Design review of the part built by this model. Coordinates are the model's own, in mm. Face numbers are marked on the shaded views. A direction names the side the tool comes from. Give positions to 0.01 mm unless a question says otherwise; leave off trailing zeros. Loops run counter-clockwise (first coordinate to the right, second up) from the corner with the lowest first, then second, coordinate; pieces in that order, holes last.
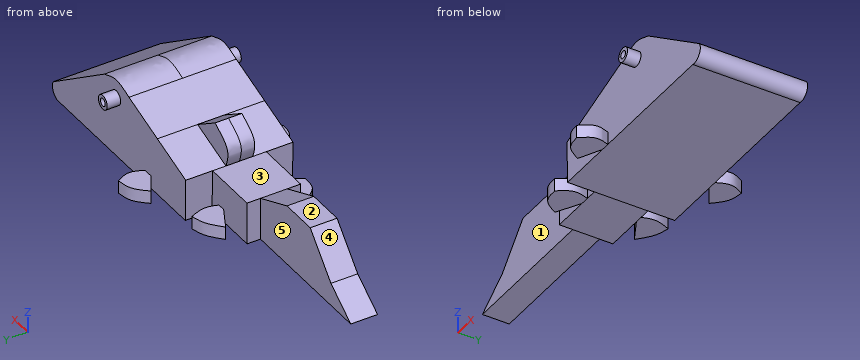
from build123d import *

# Parameters (mm, degrees)
F0_R     = 0.8499357061
F1_DEPTH = 6.35
F2_DEPTH = 3.175
F3_DEPTH = 1.5875
F4_DEPTH = 1.5875
F0_R_2   = 0.4591365961
F5_DEPTH = 7.9375
F6_DEPTH = 6.35
F9_DEPTH = 1.524


with BuildPart() as f1:
    # F0 (on Front) → F1 (new body, symmetric)
    with BuildSketch(Plane.XZ):
        with BuildLine():
            Line((3.7369009076, -7.1760629105), (27.8668981838, -7.1645976751))
            ThreePointArc((27.8668981838, -7.1645976751), (29.0924289966, -6.6745059956), (29.1452982829, -5.3556730016))
            Line((29.1452982829, -5.3556730016), (19.3140551537, 1.5164437805))
            add(Edge.make_bspline(
                [(19.3140551537, 1.5164437805), (18.5598178705, 1.842624393), (17.0255294285, 2.5061492361), (15.3991179845, 1.8500253214), (14.5722303488, 1.5164437805)],
                knots=[0, 0, 0, 0, 0.4915876753, 1, 1, 1, 1], degree=3))
            Line((14.5722303488, 1.5164437805), (9.1069049254, -0.31865054))
            Line((9.1069049254, -0.31865054), (3.641579502, -2.1537448606))
            Line((3.641579502, -2.1537448606), (3.7369009076, -7.1760629105))
        make_face()
        with Locations((17.0290809923, 0)):
            Circle(F0_R, mode=Mode.SUBTRACT)
    extrude(amount=F1_DEPTH, both=True)

    # F0 (on Front) → F2 (join, symmetric)
    with BuildSketch(Plane.XZ):
        Polygon((-3.0088014841, -7.1792680938), (3.7369009076, -7.1760629105), (3.641579502, -2.1537448606), (-2.9932308073, -2.1537448606), align=None)
    extrude(amount=F2_DEPTH, both=True)

    # F0 (on Front) → F3 (join, symmetric)
    with BuildSketch(Plane.XZ):
        Polygon((-20.3930963686, -7.1875281459), (-3.0088014841, -7.1792680938), (-2.9932308073, -2.1537448606), (-8.1067462721, 0), (-12.5872229892, 0), (-16.5754726262, -4.4647546742), align=None)
    extrude(amount=F3_DEPTH, both=True)

    # F0 (on Front) → F4 (join, symmetric)
    with BuildSketch(Plane.XZ):
        with BuildLine():
            add(Edge.make_bspline(
                [(5.739697431, 1.9025673836), (4.7061257381, 1.3267304785), (2.7990985393, 0.2642627845), (3.3769243884, -1.3941566443), (3.641579502, -2.1537448606)],
                knots=[0, 0, 0, 0, 0.5419806321, 1, 1, 1, 1], degree=3))
            Line((3.641579502, -2.1537448606), (9.1069049254, -0.31865054))
            Line((9.1069049254, -0.31865054), (5.739697431, 1.9025673836))
        make_face()
    extrude(amount=F4_DEPTH, both=True)

    # F0 (on Front) → F5 (join, symmetric)
    with BuildSketch(Plane.XZ):
        with Locations((17.0290809923, 0)):
            Circle(F0_R)
        with Locations((17.0290809923, 0)):
            Circle(F0_R_2, mode=Mode.SUBTRACT)
    extrude(amount=F5_DEPTH, both=True)

    # F0 (on Front) → F6 (join, symmetric)
    with BuildSketch(Plane.XZ):
        with Locations((17.0290809923, 0)):
            Circle(F0_R_2)
    extrude(amount=F6_DEPTH, both=True)

    # F8 (on offset) → F9 (join)
    with BuildSketch(Plane(origin=(0.0034105097, 0, -7.1778368579), x_dir=(0.9999998871, 0, 0.0004751444), z_dir=(0.0004751444, 0, -0.9999998871))):
        with BuildLine():
            Line((10.5719827116, 6.2902872451), (11.4731285721, 6.2886215746))
            add(Edge.make_bspline(
                [(11.4731285721, 6.2886215746), (11.6881530578, 6.8505612185), (12.1330545046, 8.0132553954), (11.2921062686, 9.0884414112), (10.8575951308, 9.6439812332)],
                knots=[0, 0, 0, 0, 0.483308128, 1, 1, 1, 1], degree=3))
            add(Edge.make_bspline(
                [(10.8575951308, 9.6439812332), (10.2459421425, 9.6264263255), (8.9601619026, 9.5895234992), (8.2060067921, 8.3258092197), (7.8106075525, 7.6632509008)],
                knots=[0, 0, 0, 0, 0.4757056489, 1, 1, 1, 1], degree=3))
            Line((7.8106075525, 7.6632509008), (10.5719827116, 6.2902872451))
        make_face()
        with BuildLine():
            add(Edge.make_bspline(
                [(11.445928365, -6.2551540323), (11.7208028901, -6.8377598255), (12.2652189582, -7.9916679237), (11.6289449799, -9.0578690758), (11.3139245659, -9.5857474953)],
                knots=[0, 0, 0, 0, 0.5048979368, 1, 1, 1, 1], degree=3))
            Line((11.445928365, -6.2551540323), (10.5652892962, -6.2281796709))
            Line((10.5652892962, -6.2281796709), (8.0862324685, -7.7491207048))
            add(Edge.make_bspline(
                [(11.3139245659, -9.5857474953), (10.7293926361, -9.5187590976), (9.5019236971, -9.3780889543), (8.572864944, -8.3090653448), (8.0862324685, -7.7491207048)],
                knots=[0, 0, 0, 0, 0.4762091973, 1, 1, 1, 1], degree=3))
        make_face()
        with BuildLine():
            add(Edge.make_bspline(
                [(2.4012238719, -3.135364037), (2.5766554897, -3.6317241258), (2.9495824062, -4.6868706955), (2.4212189682, -5.9031792319), (2.1414074581, -6.5473141149)],
                knots=[0, 0, 0, 0, 0.4704182467, 1, 1, 1, 1], degree=3))
            Line((2.4012238719, -3.135364037), (1.5678445343, -3.1441783067))
            Line((1.5678445343, -3.1441783067), (-1.2165163644, -4.6103880741))
            add(Edge.make_bspline(
                [(2.1414074581, -6.5473141149), (1.5835583581, -6.4193566225), (0.3958954029, -6.1469346133), (-0.6577640532, -5.1428505543), (-1.2165163644, -4.6103880741)],
                knots=[0, 0, 0, 0, 0.4697032587, 1, 1, 1, 1], degree=3))
        make_face()
        with BuildLine():
            Line((1.3515800238, 3.1687226146), (2.3737214506, 3.1360480934))
            add(Edge.make_bspline(
                [(2.3737214506, 3.1360480934), (2.5897819708, 3.7493472374), (3.0287531003, 4.9953902449), (2.2088825996, 6.1050612637), (1.792550087, 6.6685550846)],
                knots=[0, 0, 0, 0, 0.4921974706, 1, 1, 1, 1], degree=3))
            add(Edge.make_bspline(
                [(1.792550087, 6.6685550846), (1.1529153889, 6.6804914863), (-0.1895757498, 6.7055440354), (-0.9754613011, 5.3946395707), (-1.3869088143, 4.7083199024)],
                knots=[0, 0, 0, 0, 0.4764535334, 1, 1, 1, 1], degree=3))
            Line((-1.3869088143, 4.7083199024), (1.3515800238, 3.1687226146))
        make_face()
    extrude(amount=-F9_DEPTH)


solid = f1.part
Q1. Tool access review of the marked faces 1 and 2: name each direction out of +Z, -Z, +X, -X, +Y, -Y from which nothing blocks a thin tool from reaching the whole face with its end or side.
Results:
face 1: +Z, -Z, -X, -Y
face 2: +Z, -X, +Y, -Y
Q2. Take a section at B-B (x = 21.5). Give the boundary of the cut face in (y, z).
Results:
outline: (-6.35, -7.17) - (6.35, -7.17) - (6.35, -0.01) - (-6.35, -0.01) - close
Q3. Draft analysis for pull direction X (two halves, no side actions). For the marked faces 3, 4 and 5, state which applies: pulls with the +X half, pulls with the -X half, needs draft (parallel to the pull), parting line crosses it, or undercut.
Results:
face 3: undercut
face 4: pulls with the -X half
face 5: needs draft
Q4. Insertion check: pin 1 (4 mm diameter, centred on x = 2.5, z = -4, fed in from -Y); pin 2 (5 mm diameter, centred on x = 15.5, z = -2, fed in from +Y); pin 3 (3 mm diameter, centred on x = 7, z = 0.5, fed in from -Y). Each pin has a flat end and moves straight along its axis. Give the tip position at first contact, or say it passes through.
Results:
pin 1: stops at y = -6.67
pin 2: stops at y = 7.94
pin 3: stops at y = -6.35
Q5. Wall thickness on line 1 (Z direction, x = 11, y = 8.5); line 2 (Y direction, x = -17, z = -5.5); line 3 (Z direction, x = 1, y = 5.5): over which ranges is each line inside the solid? List them lowest first.
Results:
line 1: z = -7.17 to -5.65
line 2: y = -1.59 to 1.59
line 3: z = -7.18 to -5.65
Q6. Take a section at A-A (x = -5). Give the boundary of the cut face in (y, z), plus the area to 3 significant figures.
Results:
outline: (-1.59, -7.18) - (1.59, -7.18) - (1.59, -1.31) - (-1.59, -1.31) - close
area: 18.6 mm2
